Check sheet for the modelled part. Datum: model origin and axes. Units: mm. Round coordinates to 2 decimals unless told otherwise and drop trailing zeros. Write each loop counter-clockwise with the first axis right and the second up, starting at its lowest first coordinate (ties: lowest second). Pieces come first, ordered by that corner, then holes. Notation, with made-up numbers: (76.5, 74) -> (98.5, 74) arc R15 ccw to (98.5, 83) -> close; hole circle Ø9 at (-20, 41). An arc over 180 degrees is marked (long way). One line per item, written item: value. Start each with the question number.
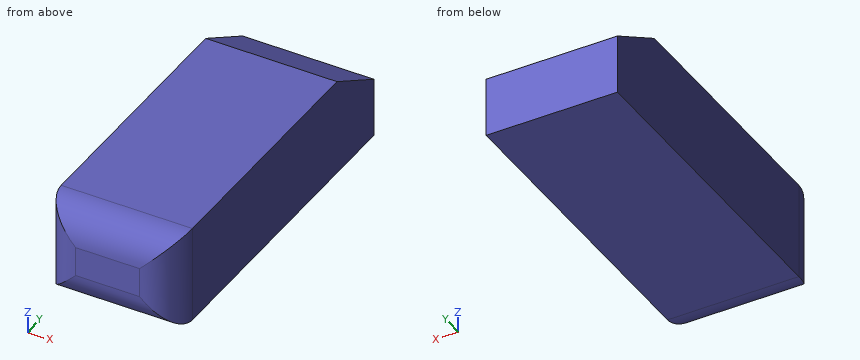
```python
from build123d import *

# Parameters (mm, degrees)
F2_DEPTH = 168.75
F3_R     = 86.75


with BuildPart() as f2:
    # F1 (on Right) → F2 (new body, symmetric)
    with BuildSketch(Plane.YZ):
        Polygon((0, 293.4), (0, 43.4), (906.2, 43.4), (906.2, 197.05), (739.3169046907, 293.4), align=None)
    extrude(amount=F2_DEPTH, both=True)

    # F3
    f3_edges = [f2.edges().sort_by_distance(p)[0] for p in [
        (0, 0, 293.4),
        (168.75, 0, 168.4),
        (-168.75, 0, 168.4),
        (0, 0, 43.4),
    ]]
    fillet(f3_edges, radius=F3_R)


solid = f2.part
```
1. Cross-section at B-B (z = 240). Record the cut outline in (x, y), plus the area to 3 significant figures.
2. Cross-section at C-C (y = 66.5). Record the cut outline in (x, z), plus the area to 3 significant figures.
3. Cross-section at A-A (x = 34.5). Record the cut outline in (y, z), plus the area to 3 significant figures.
4. Depth check by flat-ended pin: pin 1 Ø1 at (x, z) = (116, 88.5) entering from -Y; pin 2 Ø2 at (x, z) = (39.5, 99.5) entering from -Y; pin 3 Ø4 at (x, z) = (4, 108.5) entering from -Y. Enter the tip coordinate at first touch or a pass-through.
5. Material ranges on probe 1 along Y at (x, z) = (-65, 81); probe 2 along Y at (x, z) = (-130.5, 195.5); probe 3 along Z at (x, y) = (122, 769), recorded low to high.
6. Cross-section at D-D (z = 87.5). Record the cut outline in (x, y).
Working result:
1. outline: (-168.75, 86.75) arc R86.75 ccw to (-115.35, 6.67) -> (115.35, 6.67) arc R86.75 ccw to (168.75, 86.75) -> (168.75, 831.81) -> (-168.75, 831.81) -> close
1. area: 276,000 mm^2
2. outline: (-166.35, 45.8) -> (166.35, 45.8) -> (166.35, 291) -> (-166.35, 291) -> close
2. area: 81,600 mm^2
3. outline: (0, 130.15) arc R86.75 ccw to (86.75, 43.4) -> (906.2, 43.4) -> (906.2, 197.05) -> (739.32, 293.4) -> (86.75, 293.4) arc R86.75 ccw to (0, 206.65) -> close
3. area: 215,000 mm^2
4. pin 1: stops at y = 10.38
4. pin 2: stops at y = 5.22
4. pin 3: stops at y = 2.25
5. probe 1: y = 15.27 to 906.2
5. probe 2: y = 14.82 to 906.2
5. probe 3: z = 43.4 to 276.26
6. outline: (-168.75, 86.75) arc R86.75 ccw to (-124.65, 11.21) -> (124.65, 11.21) arc R86.75 ccw to (168.75, 86.75) -> (168.75, 906.2) -> (-168.75, 906.2) -> close
